from build123d import *

# Parameters (mm, degrees)
F1_DEPTH = 25
F2_SIZE  = 5
F3_R     = 5
F4_R     = 25
F5_R     = 7.049752
F6_DEPTH = 25


with BuildPart() as f1:
    # F0 (on Front) → F1 (new body)
    with BuildSketch(Plane.XZ):
        Polygon((0, 0), (30.081257, 23.027755), (29.043972, 62.029697), (-43.566033, 31.94841), align=None)
    extrude(amount=F1_DEPTH)

    # F2
    f2_edges = [f1.edges().sort_by_distance(p)[0] for p in [
        (-43.566033, -12.5, 31.94841),
    ]]
    chamfer(f2_edges, length=F2_SIZE)

    # F3
    f3_edges = [f1.edges().sort_by_distance(p)[0] for p in [
        (29.043972, -12.5, 62.029697),
    ]]
    fillet(f3_edges, radius=F3_R)

    # F4
    f4_edges = [f1.edges().sort_by_distance(p)[0] for p in [
        (30.081257, -12.5, 23.027755),
    ]]
    fillet(f4_edges, radius=F4_R)

    # F5 (on face) → F6 (join)
    with BuildSketch(Plane.XZ.offset(25)):
        with Locations((0, 40.225446)):
            Circle(F5_R)
    extrude(amount=-F6_DEPTH)


solid = f1.part
Part model, mm, in its own coordinate system. Give positions to 0.01 mm unless a question says otherwise; leave off trailing zeros. Loops run counter-clockwise (first coordinate to the right, second up) from the corner with the lowest first, then second, coordinate; pieces in that order, holes last. Notation, with made-up numbers: M -29,41.25 L -24,41.25 A5 cw -24,47.25 Z; hole C 25.25,7.25 d6. An arc over 180 degrees is marked long. Put each result on its own line as item: value. Start each with the question number.
1) Saw through at C-C (x = 16). List the corners of the cut face in (y, z).
2) Flat gauge pins, fed straight in: pin 1 (5 mm diameter, centred on x = -15, y = -5, fed in from +Z); pin 2 (3 mm diameter, centred on x = -17, y = -11.5, fed in from +Z); pin 3 (1.5 mm diameter, centred on y = -16, z = 48, fed in from +X). Where does each tip first touch, or does it go through?
3) Saw through at A-A (y = -15). List the corners of the cut face in (x, z).
4) Probe probe 1 along X at (y, z) = (-2, 37); probe 2 along Z at (x, y) = (3.5, -6); probe 3 along Z at (x, y) = (2, -20.5). List the from-to ranges inside material, lowest first.
5) Saw through at B-B (z = 4.5). List the corners of the cut face in (x, y), then the cut area to 3 significant figures.
Numbers:
1. outline: M -25,12.25 L 0,12.25 L 0,56.63 L -25,56.63 Z
2. pin 1: z = 44.82
2. pin 2: z = 43.58
2. pin 3: x = 29.44
3. outline: M -39.53,28.99 L 0,0 L 19.95,15.27 A25 ccw 29.74,35.79 L 29.24,54.76 A5 ccw 22.33,59.25 L -38.95,33.86 Z
4. probe 1: -31.37 to 29.71
4. probe 2: 2.68 to 51.45
4. probe 3: 1.53 to 50.83
5. outline: M -6.14,-25 L 5.88,-25 L 5.88,0 L -6.14,0 Z
5. area: 300 mm^2
